Geometry check sheet. Reference: the model listing, model coordinates, mm. A direction names the side the tool comes from. Round coordinates to 2 decimals unless told otherwise and drop trailing zeros. Write each loop counter-clockwise with the first axis right and the second up, starting at its lowest first coordinate (ties: lowest second). Pieces come first, ordered by that corner, then holes. Notation, with made-up numbers: (46.25, 54.5) - (104.25, 54.5) arc R19 cw to (104.25, 88.5) - close; hole circle Ø1 at (-18.5, 86). An arc over 180 degrees is marked (long way). Return JSON: item names as keys, results as strings.
```python
from build123d import *

# Parameters (mm, degrees)
SKETCH_1_R          = 5.05
SKETCH_1_R_2        = 9.5
EXTRUDE_1_DEPTH     = 12
FILLET_1_R          = 3
SKETCH_7_R          = 2.05
CUT_EXTRUDE_4_DEPTH = 277.39464539
EXTRUDE_6_DEPTH     = 12
SKETCH_8_R          = 13
CUT_EXTRUDE_5_DEPTH = 277.39464539
SKETCH_9_R          = 25
SKETCH_9_R_2        = 13
EXTRUDE_4_DEPTH     = 12
SKETCH_10_R         = 1.5
SKETCH_10_R_2       = 21.5
EXTRUDE_5_DEPTH     = 12
SKETCH_13_R         = 1.5
SKETCH_13_R_2       = 19.999997197
SKETCH_13_R_3       = 13
CUT_EXTRUDE_6_DEPTH = 25


with BuildPart() as part:
    # 草图1 → 凸台-拉伸1 (new body)
    with BuildSketch(Plane(origin=(0, 0, 0), x_dir=(1, 0, 0), z_dir=(0, 1, 0))):
        with BuildLine():
            Line((-17.992942616, -0.504), (-24.990198078, 249.3))
            ThreePointArc((-24.990198078, 249.3), (0, 275), (24.990198078, 249.3))
            Line((24.990198078, 249.3), (17.992942616, -0.504))
            ThreePointArc((17.992942616, -0.504), (0, -18), (-17.992942616, -0.504))
        make_face()
        with Locations(Location((0, 0, 0), (0, 0, 270))):
            Circle(SKETCH_1_R, mode=Mode.SUBTRACT)
        with Locations(Location((0, 250, 0), (0, 0, 270))):
            Circle(SKETCH_1_R_2, mode=Mode.SUBTRACT)
        Polygon((-16.444447487, 158.5), (-17.704941698, 203.5), (11.028871219, 137.174942267), align=None, mode=Mode.SUBTRACT)
        Polygon((15.954255294, 141), (18.475243716, 231), (-12, 219.5), align=None, mode=Mode.SUBTRACT)
    extrude(amount=EXTRUDE_1_DEPTH)

    # 圆角1
    fillet_1_edges = [part.edges().sort_by_distance(p)[0] for p in [
        (-16.444447487, 6, -158.5),
        (11.028871219, 6, -137.174942267),
        (-17.704941698, 6, -203.5),
        (18.475243716, 6, -231),
        (-12, 6, -219.5),
        (15.954255294, 6, -141),
    ]]
    fillet(fillet_1_edges, radius=FILLET_1_R)

    # 草图7 → 切除-拉伸4 (cut, through all)
    with BuildSketch(Plane(origin=(0, 12, 0), x_dir=(1, 0, 0), z_dir=(0, 1, 0))):
        with Locations(Location((15, 15, 0), (0, 0, 270))):
            Circle(SKETCH_7_R)
        with Locations(Location((-15, 15, 0), (0, 0, 270))):
            Circle(SKETCH_7_R)
        with Locations((-15, -15)):
            Circle(SKETCH_7_R)
        with Locations((15, -15)):
            Circle(SKETCH_7_R)
    extrude(amount=-CUT_EXTRUDE_4_DEPTH, mode=Mode.SUBTRACT)

    # 草图14 → 凸台-拉伸6 (add)
    with BuildSketch(Plane(origin=(0, 12, 0), x_dir=(1, 0, 0), z_dir=(0, 1, 0))):
        Polygon((-17.958821841, 235.186562879), (21.367198419, 232.917754018), (15.538653821, 131.889647666), (-22.497275836, 156.52002696), align=None)
    extrude(amount=-EXTRUDE_6_DEPTH)

    # 草图8 → 切除-拉伸5 (cut, through all)
    with BuildSketch(Plane(origin=(0, 12, 0), x_dir=(1, 0, 0), z_dir=(0, 1, 0))):
        with Locations(Location((0, 0, 0), (0, 0, 270))):
            Circle(SKETCH_8_R)
    extrude(amount=-CUT_EXTRUDE_5_DEPTH, mode=Mode.SUBTRACT)

    # 草图9 → 凸台-拉伸4 (add)
    with BuildSketch(Plane(origin=(0, 12, 0), x_dir=(1, 0, 0), z_dir=(0, 1, 0))):
        Circle(SKETCH_9_R)
        with Locations(Location((0, 0, 0), (0, 0, 270))):
            Circle(SKETCH_9_R_2, mode=Mode.SUBTRACT)
    extrude(amount=-EXTRUDE_4_DEPTH)

    # 草图10 → 凸台-拉伸5 (add)
    with BuildSketch(Plane(origin=(0, 12, 0), x_dir=(1, 0, 0), z_dir=(0, 1, 0))):
        with BuildLine():
            Line((-39.711049207, 4.799226071), (-40, 0))
            ThreePointArc((-40, 0), (0, -40), (40, 0))
            Line((40, 0), (39.711049207, 4.799226071))
            Line((39.711049207, 4.799226071), (24.990198078, 249.3))
            Line((24.990198078, 249.3), (18.993134598, 35.203136766))
            ThreePointArc((18.993134598, 35.203136766), (0, 40), (-18.993134598, 35.203136766))
            Line((-18.993134598, 35.203136766), (-24.990198078, 249.3))
            Line((-24.990198078, 249.3), (-39.711049207, 4.799226071))
        make_face()
        with Locations(Location((-31.493406412, -20.357194124, 0), (0, 0, 270))):
            Circle(SKETCH_10_R, mode=Mode.SUBTRACT)
        with Locations(Location((-37.210701127, 4.649055992, 0), (0, 0, 270))):
            Circle(SKETCH_10_R, mode=Mode.SUBTRACT)
        with Locations(Location((-11.039996826, -35.838086864, 0), (0, 0, 270))):
            Circle(SKETCH_10_R, mode=Mode.SUBTRACT)
        with Locations((-1.883144055, 37.452687066)):
            Circle(SKETCH_10_R, mode=Mode.SUBTRACT)
        with Locations(Location((14.579149971, -34.549940465, 0), (0, 0, 270))):
            Circle(SKETCH_10_R, mode=Mode.SUBTRACT)
        Circle(SKETCH_10_R_2, mode=Mode.SUBTRACT)
        with Locations(Location((33.376550467, -17.095492942, 0), (0, 0, 270))):
            Circle(SKETCH_10_R, mode=Mode.SUBTRACT)
        with Locations(Location((36.55669206, 8.358125723, 0), (0, 0, 270))):
            Circle(SKETCH_10_R, mode=Mode.SUBTRACT)
    extrude(amount=-EXTRUDE_5_DEPTH)

    # 草图13 → 切除-拉伸6 (cut)
    # profile 1 of 3: a face of its own
    with BuildSketch(Plane(origin=(0, 12, 0), x_dir=(1, 0, 0), z_dir=(0, 1, 0))):
        with BuildLine():
            ThreePointArc((-40, 0), (0, -40), (40, 0))
            Line((40, 0), (24.990198078, 249.3))
            ThreePointArc((24.990198078, 249.3), (0, 275), (-24.990198078, 249.3))
            Line((-24.990198078, 249.3), (-40, 0))
        make_face()
        with Locations((-31.493406412, -20.357194124)):
            Circle(SKETCH_13_R, mode=Mode.SUBTRACT)
        with Locations((-37.210701127, 4.649055992)):
            Circle(SKETCH_13_R, mode=Mode.SUBTRACT)
        with Locations((-11.039996826, -35.838086864)):
            Circle(SKETCH_13_R, mode=Mode.SUBTRACT)
        with Locations((14.579149971, -34.549940465)):
            Circle(SKETCH_13_R, mode=Mode.SUBTRACT)
        with Locations((33.376550467, -17.095492942)):
            Circle(SKETCH_13_R, mode=Mode.SUBTRACT)
        with Locations((36.55669206, 8.358125723)):
            Circle(SKETCH_13_R, mode=Mode.SUBTRACT)
        with BuildLine():
            ThreePointArc((-28.327815251, 9.875975047), (-25.64448638, 19.916210003), (-24.477251587, 30.243074713))
            Line((-24.477251587, 30.243074713), (-17.051673854, 224.281506908))
            ThreePointArc((-17.051673854, 224.281506908), (-17.426051547, 234.665479827), (-19.333438467, 244.879633115))
            ThreePointArc((-19.333438467, 244.879633115), (0, 270), (19.333438467, 244.879633115))
            ThreePointArc((19.333438467, 244.879633115), (17.426051547, 234.665479827), (17.051673854, 224.281506908))
            Line((17.051673854, 224.281506908), (24.477251587, 30.243074713))
            ThreePointArc((24.477251587, 30.243074713), (25.64448638, 19.916210003), (28.327815251, 9.875975047))
            ThreePointArc((28.327815251, 9.875975047), (0, -30), (-28.327815251, 9.875975047))
        make_face(mode=Mode.SUBTRACT)
    # profile 2 of 3: a face of its own
    with BuildSketch(Plane(origin=(0, 12, 0), x_dir=(1, 0, 0), z_dir=(0, 1, 0))):
        with BuildLine():
            ThreePointArc((6, 200), (0, 206), (-6, 200))
            Line((-6, 200), (-10, 50))
            ThreePointArc((-10, 50), (0, 40), (10, 50))
            Line((10, 50), (6, 200))
        make_face()
    # profile 3 of 3: a face of its own
    with BuildSketch(Plane(origin=(0, 12, 0), x_dir=(1, 0, 0), z_dir=(0, 1, 0))):
        with Locations(Location((0, 0, 0), (0, 0, 270))):
            Circle(SKETCH_13_R_2)
        Circle(SKETCH_13_R_3, mode=Mode.SUBTRACT)
    extrude(amount=-CUT_EXTRUDE_6_DEPTH, mode=Mode.SUBTRACT)


solid = part.part
```
(1) Material ranges on line 1 along X through (y, z) = (8.75, -172); line 2 along X through (y, z) = (2.5, -250); line 3 along Z through (x, y) = (2, 1.25), recorded low to high. Write a range as [from, to].
Response values:
{"line 1": "x = [-19.05, -6.75], [6.75, 19.05]", "line 2": "x = [-20, -9.5], [9.5, 20]", "line 3": "z = [-269.9, -259.29], [-240.71, -205.66], [-40.2, -19.9], [19.9, 29.93]"}
(2) Section check A-A, the plane y = 3.5. Enter the section's corners in (x, z), plus the area to 3 significant figures.
Response values:
{"outline": "(-28.33, -9.88) arc R70 cw to (-24.48, -30.24) - (-17.05, -224.28) arc R70 cw to (-19.33, -244.88) arc R20 ccw (long way) to (19.33, -244.88) arc R70 cw to (17.05, -224.28) - (24.48, -30.24) arc R70 cw to (28.33, -9.88) arc R30 ccw (long way) to start; hole circle Ø40 at (0, 0); hole (-10, -50) - (-6, -200) arc R6 ccw to (6, -200) - (10, -50) arc R10 ccw to start; hole circle Ø19 at (0, -250)", "area": "8,510 mm^2"}
(3) Section check D-D, the plane z = 0. Enter the section's corners in (x, y).
Response values:
{"outline": "(-30, 0) - (-20, 0) - (-20, 12) - (-30, 12) - close; (20, 0) - (30, 0) - (30, 12) - (20, 12) - close"}
(4) Access from +Z, -Z, +X, -X, +Y, -Y to the whole of each face (thin tool, end or side, straight path). Record for faces 1 (the face through (0, 6, -40)), 2 (the face through (-17.41, 6.08, -234.52)), 3 (the face through (20.712, 6.084, -128.621)), 4 (the face through (13, 12, -122)).
Response values:
{"face 1": "+Y, -Y", "face 2": "-X, +Y, -Y", "face 3": "+X, +Y, -Y", "face 4": "+Z, -Z, +X, -X, +Y"}
(5) Release check for a two-part mould opening along Z. For faces 5 (the face through (13, 0, -122)), 6 (the face through (0.8, 6.08, 29.99)), 7 (the face through (-20.816, 6.084, -125.904)), 8 (the face through (0, 6, -206)) record: pulls with the +Z half, pulls with the -Z half, needs draft (parallel to the pull), parting line crosses it, or undercut.
Response values:
{"face 5": "needs draft", "face 6": "parting line crosses it", "face 7": "undercut", "face 8": "undercut"}
(6) Gauge pin test, flat ends, axial feed: pin 1 (2 mm diameter, centred on y = 9, z = -219, fed in from +X); pin 2 (1.5 mm diameter, centred on y = 5, z = -156.5, fed in from +X); pin 3 (3 mm diameter, centred on y = 6.5, z = -239, fed in from +X); pin 4 (8 mm diameter, centred on x = 23, z = -220.5, fed in from -Y). Record the tip position at first contact, or that the pin passes through.
Response values:
{"pin 1": "stops at x = 17.29", "pin 2": "stops at x = 19.67", "pin 3": "stops at x = 18.32", "pin 4": "passes through"}
(7) Section check C-C, the plane x = 0. Enter the section's corners in (y, z), plus the area to 3 significant figures.
Response values:
{"outline": "(0, -270) - (12, -270) - (12, -259.5) - (0, -259.5) - close; (0, -240.5) - (12, -240.5) - (12, -206) - (0, -206) - close; (0, -40) - (12, -40) - (12, -20) - (0, -20) - close; (0, 20) - (12, 20) - (12, 30) - (0, 30) - close", "area": "900 mm^2"}
(8) Section check B-B, the plane z = -250. Enter the section's corners in (x, y), plus the area to 3 significant figures.
Response values:
{"outline": "(-20, 0) - (-9.5, 0) - (-9.5, 12) - (-20, 12) - close; (9.5, 0) - (20, 0) - (20, 12) - (9.5, 12) - close", "area": "252 mm^2"}
